from build123d import *

# Parameters (mm, degrees)
F0_W            = 10
F0_H            = 17.5
F3_D            = 6
F4_T            = -2
F6_D            = 8
F6_COPIES_COUNT = 5
F7_SIZE         = 1


# Not quite as in the source:
# - a pattern or mirror of a feature is missing from the dataset's text; its kind, count and spacing are read off the source's solid


with BuildPart() as f1:
    # F0 (on Front) → F1 (revolve)
    with BuildSketch(Plane.XZ):
        with Locations((5, 8.75)):
            Rectangle(F0_W, F0_H)
    revolve(axis=Axis((5, 0, 0), (1, 0, 0)))

    # F3 (through all)
    with Locations(Plane(origin=(0, 0, 0), x_dir=(0, 1, 0), z_dir=(-1, 0, 0))):
        with Locations((0, 0)):
            Hole(F3_D / 2)

    # F4
    f4_openings = [f1.faces().sort_by_distance(p)[0] for p in [
        (10, 0, -17.005025),
    ]]
    offset(amount=F4_T, openings=f4_openings)

    # F6 (through all)
    with Locations(Plane(origin=(0, 0, 0), x_dir=(0, -1, 0), z_dir=(-1, 0, 0))):
        with Locations((0, 10)):
            f6 = Hole(F6_D / 2)

    # F6_copies: F6 ×5 about axis
    f6_copies_axis = Axis((0, 0, 0), (1, 0, 0))
    for i in range(1, F6_COPIES_COUNT):
        add(f6.rotate(f6_copies_axis, i * 360 / F6_COPIES_COUNT), mode=Mode.SUBTRACT)

    # F7
    f7_edges = [f1.edges().sort_by_distance(p)[0] for p in [
        (10, -5, 0),
    ]]
    chamfer(f7_edges, length=F7_SIZE)


solid = f1.part
Work out the finished part from the listing and answer in its coordinate system (mm). A direction names the side the tool comes from. Give positions to 0.01 mm unless a question says otherwise; leave off trailing zeros. Write each loop counter-clockwise with the first axis right and the second up, starting at its lowest first coordinate (ties: lowest second). Pieces come first, ordered by that corner, then holes. Notation, with made-up numbers: (66.25, -23) - (77.25, -23) arc R13 ccw to (77.25, -2) - close; hole circle Ø6 at (5.5, 57). An arc over 180 degrees is marked (long way). One line per item, written item: value. Start each with the question number.
1. Find section D-D (y = 13). Write down the section's boundary in (x, z).
2. Find section C-C (x = 8). Write down the section's boundary in (y, z), then the cut area to 3 significant figures.
3. For faces 1 (the cylindrical face through (1, 2.3, -6.3)), 2 (the cylindrical face through (6.056, -15.368, -2.018)), determine the directions among +Z, -Z, +X, -X, +Y, -Y from which every point of the face is accessible in a straight line to the end or side of a thin tool.
4. Find section B-B (z = 8). Write down the section's boundary in (x, y).
5. Consider probe 1 along Z at (x, y) = (7, 0); probe 2 along Y at (x, z) = (6, -2); probe 3 along Z at (x, y) = (2.25, -3.5). Determine where each line is inside the solid, lowest interval first.
6. For a pull along Y with two mould halves and no side action, classify faces 3 (the cylindrical face through (5.07, 10.648, -13.887)), 4 (the flat face through (10, -3, -1)), 5 (the cylindrical face through (1.01, -5.08, -12.01)) as +Y half, -Y half, draft (parallel to the pull), parting line (faces both ways), or undercut.
7. Find section A-A (y = 0). Write down the section's boundary in (x, z).
8. Given pin 1 (5 mm diameter, centred on y = -9.51, z = 3.09, fed in from +X); pin 2 (5 mm diameter, centred on x = 8, z = -7.5, fed in from +Y); pin 3 (6 mm diameter, centred on x = 1.5, y = -7.5, fed in from +Z); pin 4 (10.5 mm diameter, centred on y = 5.88, z = -8.09, fed in from +X), each flat-ended and moving along its own axis, determine where each tip first touches the part or whether it passes through.
Geometry results:
1. outline: (0, -11.72) - (10, -11.72) - (10, -8.44) - (2, -8.44) - (2, 1.13) - (0, 1.13) - close; (0, 5.05) - (2, 5.05) - (2, 8.44) - (10, 8.44) - (10, 11.72) - (0, 11.72) - close
2. outline: circle Ø35 at (0, 0); circle Ø10 at (0, 0); hole circle Ø31 at (0, 0); hole circle Ø6 at (0, 0)
2. area: 258 mm2
3. face 1: +X, -X
3. face 2: +X
4. outline: (0, -15.56) - (10, -15.56) - (10, -13.28) - (2, -13.28) - (2, -3.46) - (0, -3.46) - close; (0, 3.46) - (2, 3.46) - (2, 13.28) - (10, 13.28) - (10, 15.56) - (0, 15.56) - close
5. probe 1: -17.5 to -15.5, -5 to -3, 3 to 5, 15.5 to 17.5
5. probe 2: -17.39 to -15.37, -4.58 to -2.24, 2.24 to 4.58, 15.37 to 17.39
5. probe 3: -17.15 to -15.1, -3.57 to 3.57, 15.1 to 17.15
6. face 3: parting line
6. face 4: draft
6. face 5: undercut
7. outline: (0, -17.5) - (10, -17.5) - (10, -15.5) - (2, -15.5) - (2, -5) - (9, -5) - (10, -4) - (10, -3) - (0, -3) - close; (0, 3) - (10, 3) - (10, 4) - (9, 5) - (2, 5) - (2, 6) - (0, 6) - close; (0, 14) - (2, 14) - (2, 15.5) - (10, 15.5) - (10, 17.5) - (0, 17.5) - close
8. pin 1: through
8. pin 2: y = 16.77
8. pin 3: z = 16.91
8. pin 4: x = 9.25
